```python
from build123d import *

# Parameters (mm, degrees)
SKETCH2_W           = 40
SKETCH2_H           = 34
BOSS_EXTRUDE1_DEPTH = 3.75
SKETCH3_W           = 49.149
SKETCH3_H           = 41.783
BOSS_EXTRUDE2_DEPTH = 1.016
CUT_EXTRUDE1_REACH  = 34.524
SKETCH4_R           = 1.6383
FILLET1_R           = 2.159
CUT_EXTRUDE2_REACH  = 34.524
SKETCH5_R           = 0.649719702
SKETCH6_W           = 36
SKETCH6_H           = 26
CUT_EXTRUDE3_DEPTH  = 0.1016
FILLET2_R           = 3
FILLET3_R           = 1
FILLET4_R           = 1


with BuildPart() as part:
    # Sketch2 → Boss-Extrude1 (new body)
    with BuildSketch(Plane(origin=(0, 0, 0), x_dir=(1, 0, 0), z_dir=(0, 1, 0))):
        Rectangle(SKETCH2_W, SKETCH2_H)
    extrude(amount=BOSS_EXTRUDE1_DEPTH)

    # Sketch3 → Boss-Extrude2 (add)
    with BuildSketch(Plane(origin=(0, 0, 0), x_dir=(1, 0, 0), z_dir=(0, 1, 0))):
        with Locations((0, -0.0815)):
            Rectangle(SKETCH3_W, SKETCH3_H)
    extrude(amount=-BOSS_EXTRUDE2_DEPTH)

    # Sketch4 → Cut-Extrude1 (cut, up to next)
    with BuildSketch(Plane(origin=(0, 0, 0), x_dir=(1, 0, 0), z_dir=(0, 1, 0)), mode=Mode.PRIVATE) as cut_extrude1_sk1:
        with Locations(Location((-22.5, 18.5, 0), (0, 0, 270))):
            Circle(SKETCH4_R)
    cut_extrude1_tool1 = extrude(cut_extrude1_sk1.sketch, amount=-CUT_EXTRUDE1_REACH, mode=Mode.PRIVATE) & part.part
    # Sketch4 → Cut-Extrude1 (cut, up to next)
    with BuildSketch(Plane(origin=(0, 0, 0), x_dir=(1, 0, 0), z_dir=(0, 1, 0)), mode=Mode.PRIVATE) as cut_extrude1_sk2:
        with Locations(Location((-22.5, -18.5, 0), (0, 0, 270))):
            Circle(SKETCH4_R)
    cut_extrude1_tool2 = extrude(cut_extrude1_sk2.sketch, amount=-CUT_EXTRUDE1_REACH, mode=Mode.PRIVATE) & part.part
    # Sketch4 → Cut-Extrude1 (cut, up to next)
    with BuildSketch(Plane(origin=(0, 0, 0), x_dir=(1, 0, 0), z_dir=(0, 1, 0)), mode=Mode.PRIVATE) as cut_extrude1_sk3:
        with Locations(Location((22.5, 18.5, 0), (0, 0, 270))):
            Circle(SKETCH4_R)
    cut_extrude1_tool3 = extrude(cut_extrude1_sk3.sketch, amount=-CUT_EXTRUDE1_REACH, mode=Mode.PRIVATE) & part.part
    # Sketch4 → Cut-Extrude1 (cut, up to next)
    with BuildSketch(Plane(origin=(0, 0, 0), x_dir=(1, 0, 0), z_dir=(0, 1, 0)), mode=Mode.PRIVATE) as cut_extrude1_sk4:
        with Locations(Location((22.5, -18.5, 0), (0, 0, 270))):
            Circle(SKETCH4_R)
    cut_extrude1_tool4 = extrude(cut_extrude1_sk4.sketch, amount=-CUT_EXTRUDE1_REACH, mode=Mode.PRIVATE) & part.part
    add(cut_extrude1_tool1.solids().sort_by_distance((-22.5, 0, -18.5))[0], mode=Mode.SUBTRACT)
    add(cut_extrude1_tool2.solids().sort_by_distance((-22.5, 0, 18.5))[0], mode=Mode.SUBTRACT)
    add(cut_extrude1_tool3.solids().sort_by_distance((22.5, 0, -18.5))[0], mode=Mode.SUBTRACT)
    add(cut_extrude1_tool4.solids().sort_by_distance((22.5, 0, 18.5))[0], mode=Mode.SUBTRACT)

    # Fillet1
    fillet1_edges = [part.edges().sort_by_distance(p)[0] for p in [
        (-24.5745, -0.508, 20.973),
        (-24.5745, -0.508, -20.81),
        (24.5745, -0.508, -20.81),
        (24.5745, -0.508, 20.973),
    ]]
    fillet(fillet1_edges, radius=FILLET1_R)

    # Sketch5 → Cut-Extrude2 (cut, up to next)
    with BuildSketch(Plane(origin=(0, 0, 0), x_dir=(1, 0, 0), z_dir=(0, 1, 0)), mode=Mode.PRIVATE) as cut_extrude2_sk1:
        with Locations(Location((-1.27, 19.2225, 0), (0, 0, 270))):
            Circle(SKETCH5_R)
    cut_extrude2_tool1 = extrude(cut_extrude2_sk1.sketch, amount=-CUT_EXTRUDE2_REACH, mode=Mode.PRIVATE) & part.part
    # Sketch5 → Cut-Extrude2 (cut, up to next)
    with BuildSketch(Plane(origin=(0, 0, 0), x_dir=(1, 0, 0), z_dir=(0, 1, 0)), mode=Mode.PRIVATE) as cut_extrude2_sk2:
        with Locations(Location((-3.81, 19.2225, 0), (0, 0, 270))):
            Circle(SKETCH5_R)
    cut_extrude2_tool2 = extrude(cut_extrude2_sk2.sketch, amount=-CUT_EXTRUDE2_REACH, mode=Mode.PRIVATE) & part.part
    # Sketch5 → Cut-Extrude2 (cut, up to next)
    with BuildSketch(Plane(origin=(0, 0, 0), x_dir=(1, 0, 0), z_dir=(0, 1, 0)), mode=Mode.PRIVATE) as cut_extrude2_sk3:
        with Locations(Location((-6.35, 19.2225, 0), (0, 0, 270))):
            Circle(SKETCH5_R)
    cut_extrude2_tool3 = extrude(cut_extrude2_sk3.sketch, amount=-CUT_EXTRUDE2_REACH, mode=Mode.PRIVATE) & part.part
    # Sketch5 → Cut-Extrude2 (cut, up to next)
    with BuildSketch(Plane(origin=(0, 0, 0), x_dir=(1, 0, 0), z_dir=(0, 1, 0)), mode=Mode.PRIVATE) as cut_extrude2_sk4:
        with Locations(Location((1.27, 19.2225, 0), (0, 0, 270))):
            Circle(SKETCH5_R)
    cut_extrude2_tool4 = extrude(cut_extrude2_sk4.sketch, amount=-CUT_EXTRUDE2_REACH, mode=Mode.PRIVATE) & part.part
    # Sketch5 → Cut-Extrude2 (cut, up to next)
    with BuildSketch(Plane(origin=(0, 0, 0), x_dir=(1, 0, 0), z_dir=(0, 1, 0)), mode=Mode.PRIVATE) as cut_extrude2_sk5:
        with Locations(Location((3.81, 19.2225, 0), (0, 0, 270))):
            Circle(SKETCH5_R)
    cut_extrude2_tool5 = extrude(cut_extrude2_sk5.sketch, amount=-CUT_EXTRUDE2_REACH, mode=Mode.PRIVATE) & part.part
    # Sketch5 → Cut-Extrude2 (cut, up to next)
    with BuildSketch(Plane(origin=(0, 0, 0), x_dir=(1, 0, 0), z_dir=(0, 1, 0)), mode=Mode.PRIVATE) as cut_extrude2_sk6:
        with Locations(Location((6.35, 19.2225, 0), (0, 0, 270))):
            Circle(SKETCH5_R)
    cut_extrude2_tool6 = extrude(cut_extrude2_sk6.sketch, amount=-CUT_EXTRUDE2_REACH, mode=Mode.PRIVATE) & part.part
    # Sketch5 → Cut-Extrude2 (cut, up to next)
    with BuildSketch(Plane(origin=(0, 0, 0), x_dir=(1, 0, 0), z_dir=(0, 1, 0)), mode=Mode.PRIVATE) as cut_extrude2_sk7:
        with Locations(Location((6.35, -18.687, 0), (0, 0, 90))):
            Circle(SKETCH5_R)
    cut_extrude2_tool7 = extrude(cut_extrude2_sk7.sketch, amount=-CUT_EXTRUDE2_REACH, mode=Mode.PRIVATE) & part.part
    # Sketch5 → Cut-Extrude2 (cut, up to next)
    with BuildSketch(Plane(origin=(0, 0, 0), x_dir=(1, 0, 0), z_dir=(0, 1, 0)), mode=Mode.PRIVATE) as cut_extrude2_sk8:
        with Locations(Location((3.81, -18.687, 0), (0, 0, 90))):
            Circle(SKETCH5_R)
    cut_extrude2_tool8 = extrude(cut_extrude2_sk8.sketch, amount=-CUT_EXTRUDE2_REACH, mode=Mode.PRIVATE) & part.part
    # Sketch5 → Cut-Extrude2 (cut, up to next)
    with BuildSketch(Plane(origin=(0, 0, 0), x_dir=(1, 0, 0), z_dir=(0, 1, 0)), mode=Mode.PRIVATE) as cut_extrude2_sk9:
        with Locations(Location((1.27, -18.687, 0), (0, 0, 90))):
            Circle(SKETCH5_R)
    cut_extrude2_tool9 = extrude(cut_extrude2_sk9.sketch, amount=-CUT_EXTRUDE2_REACH, mode=Mode.PRIVATE) & part.part
    # Sketch5 → Cut-Extrude2 (cut, up to next)
    with BuildSketch(Plane(origin=(0, 0, 0), x_dir=(1, 0, 0), z_dir=(0, 1, 0)), mode=Mode.PRIVATE) as cut_extrude2_sk10:
        with Locations(Location((-6.35, -18.687, 0), (0, 0, 90))):
            Circle(SKETCH5_R)
    cut_extrude2_tool10 = extrude(cut_extrude2_sk10.sketch, amount=-CUT_EXTRUDE2_REACH, mode=Mode.PRIVATE) & part.part
    # Sketch5 → Cut-Extrude2 (cut, up to next)
    with BuildSketch(Plane(origin=(0, 0, 0), x_dir=(1, 0, 0), z_dir=(0, 1, 0)), mode=Mode.PRIVATE) as cut_extrude2_sk11:
        with Locations(Location((-3.81, -18.687, 0), (0, 0, 90))):
            Circle(SKETCH5_R)
    cut_extrude2_tool11 = extrude(cut_extrude2_sk11.sketch, amount=-CUT_EXTRUDE2_REACH, mode=Mode.PRIVATE) & part.part
    # Sketch5 → Cut-Extrude2 (cut, up to next)
    with BuildSketch(Plane(origin=(0, 0, 0), x_dir=(1, 0, 0), z_dir=(0, 1, 0)), mode=Mode.PRIVATE) as cut_extrude2_sk12:
        with Locations(Location((-1.27, -18.687, 0), (0, 0, 90))):
            Circle(SKETCH5_R)
    cut_extrude2_tool12 = extrude(cut_extrude2_sk12.sketch, amount=-CUT_EXTRUDE2_REACH, mode=Mode.PRIVATE) & part.part
    add(cut_extrude2_tool1.solids().sort_by_distance((-1.27, 0, -19.2225))[0], mode=Mode.SUBTRACT)
    add(cut_extrude2_tool2.solids().sort_by_distance((-3.81, 0, -19.2225))[0], mode=Mode.SUBTRACT)
    add(cut_extrude2_tool3.solids().sort_by_distance((-6.35, 0, -19.2225))[0], mode=Mode.SUBTRACT)
    add(cut_extrude2_tool4.solids().sort_by_distance((1.27, 0, -19.2225))[0], mode=Mode.SUBTRACT)
    add(cut_extrude2_tool5.solids().sort_by_distance((3.81, 0, -19.2225))[0], mode=Mode.SUBTRACT)
    add(cut_extrude2_tool6.solids().sort_by_distance((6.35, 0, -19.2225))[0], mode=Mode.SUBTRACT)
    add(cut_extrude2_tool7.solids().sort_by_distance((6.35, 0, 18.687))[0], mode=Mode.SUBTRACT)
    add(cut_extrude2_tool8.solids().sort_by_distance((3.81, 0, 18.687))[0], mode=Mode.SUBTRACT)
    add(cut_extrude2_tool9.solids().sort_by_distance((1.27, 0, 18.687))[0], mode=Mode.SUBTRACT)
    add(cut_extrude2_tool10.solids().sort_by_distance((-6.35, 0, 18.687))[0], mode=Mode.SUBTRACT)
    add(cut_extrude2_tool11.solids().sort_by_distance((-3.81, 0, 18.687))[0], mode=Mode.SUBTRACT)
    add(cut_extrude2_tool12.solids().sort_by_distance((-1.27, 0, 18.687))[0], mode=Mode.SUBTRACT)

    # Sketch6 → Cut-Extrude3 (cut)
    with BuildSketch(Plane(origin=(0, 3.75, 0), x_dir=(1, 0, 0), z_dir=(0, 1, 0))):
        with Locations((0, 2.75)):
            Rectangle(SKETCH6_W, SKETCH6_H)
    extrude(amount=-CUT_EXTRUDE3_DEPTH, mode=Mode.SUBTRACT)

    # Fillet2
    fillet2_edges = [part.edges().sort_by_distance(p)[0] for p in [
        (-18, 3.6992, 10.25),
        (-18, 3.6992, -15.75),
        (18, 3.6992, -15.75),
        (18, 3.6992, 10.25),
    ]]
    fillet(fillet2_edges, radius=FILLET2_R)

    # Fillet3
    fillet3_edges = [part.edges().sort_by_distance(p)[0] for p in [
        (-20, 1.875, -17),
        (20, 1.875, -17),
        (20, 1.875, 17),
        (-20, 1.875, 17),
    ]]
    fillet(fillet3_edges, radius=FILLET3_R)

    # Fillet4
    fillet4_edges = [part.edges().sort_by_distance(p)[0] for p in [
        (-20, 3.75, 0),
        (0, 3.75, -17),
        (0, 3.75, 17),
        (20, 3.75, 0),
        (19.707106781, 3.75, -16.707106781),
        (19.707106781, 3.75, 16.707106781),
        (-19.707106781, 3.75, 16.707106781),
        (-19.707106781, 3.75, -16.707106781),
    ]]
    fillet(fillet4_edges, radius=FILLET4_R)


solid = part.part
```
Can you work these out from the model? Positions are in its coordinate system, mm. A direction names the side the tool comes from. Give positions to 0.01 mm unless a question says otherwise; leave off trailing zeros. Write each loop counter-clockwise with the first axis right and the second up, starting at its lowest first coordinate (ties: lowest second). Pieces come first, ordered by that corner, then holes. Notation, with made-up numbers: (54.25, 23.5) -> (78.25, 23.5) arc R26 ccw to (78.25, 51.5) -> close; hole circle Ø6 at (84, -17). An arc over 180 degrees is marked (long way). One line per item, written item: value.
Q1. We'd pull the mould along X, two halves only. Please class faces 4 (the face through (-0.3, -0.5, -20.81)), 5 (the face through (-23.95, -0.5, 19.26)), 6 (the face through (19.699, 3.465, 0.224)): +X half, -X half, draft (parallel to the pull), parting line (faces both ways), or undercut.
Results found:
face 4: draft
face 5: undercut
face 6: +X half
Q2. Which directions (+Z, -Z, +X, -X, +Y, -Y) give clear straight access to the entire face, cutting with the end or side of a thin tool? Please do faces 1 (the face through (20, 1, 0)), 2 (the face through (-19.715, 1.394, 16.699)), 3 (the face through (-19.715, 1.394, -16.699)).
Results found:
face 1: +Z, -Z, +X, +Y
face 2: +Z, -X, +Y
face 3: -Z, -X, +Y
Q3. Please list where these lines run through material, in increasing order: line 1 (X direction, y = -0.8, z = -18.5); line 2 (X direction, y = 1.05, z = -12.5); line 3 (Y direction, x = -7.5, z = -5). Write a range as [from, to].
Results found:
line 1: x = [-24.57, -24.14], [-20.86, 20.86], [24.14, 24.57]
line 2: x = [-20, 20]
line 3: y = [-1.02, 3.65]
Q4. Imagine slicing it at B-B on y = 1. Please give me the cut outline in (x, z), and give its area (3 significant figures).
Results found:
outline: (-20, -16) arc R1 ccw to (-19, -17) -> (19, -17) arc R1 ccw to (20, -16) -> (20, 16) arc R1 ccw to (19, 17) -> (-19, 17) arc R1 ccw to (-20, 16) -> close
area: 1,360 mm^2
Q5. Imagine slicing it at D-D on z = -11. Please give me the cut outline in (x, y), and give its area (3 significant figures).
Results found:
outline: (-24.57, -1.02) -> (24.57, -1.02) -> (24.57, 0) -> (20, 0) -> (20, 2.75) arc R1 ccw to (19, 3.75) -> (18, 3.75) -> (18, 3.65) -> (-18, 3.65) -> (-18, 3.75) -> (-19, 3.75) arc R1 ccw to (-20, 2.75) -> (-20, 0) -> (-24.57, 0) -> close
area: 196 mm^2
Q6. Imagine slicing it at A-A on x = -6.35. Please give me the cut outline in (y, z).
Results found:
outline: (-1.02, -20.81) -> (0, -20.81) -> (0, -19.87) -> (-1.02, -19.87) -> close; (-1.02, -18.57) -> (0, -18.57) -> (0, -17) -> (2.75, -17) arc R1 ccw to (3.75, -16) -> (3.75, -15.75) -> (3.65, -15.75) -> (3.65, 10.25) -> (3.75, 10.25) -> (3.75, 16) arc R1 ccw to (2.75, 17) -> (0, 17) -> (0, 18.04) -> (-1.02, 18.04) -> close; (-1.02, 19.34) -> (0, 19.34) -> (0, 20.97) -> (-1.02, 20.97) -> close
Q7. For P1, Ø1, axis at x = 5.5, z = 2, coming from the +Y side; P2, Ø1.5, axis at x = -1.27, z = -19.22, coming from the +Y side; P3, Ø2, axis at y = 1.5, z = -16.5, coming from the -X side, each with a flat end and sliding along its axis, tell me the tip position at first contact or that it passes through.
Results found:
P1: stops at y = 3.65
P2: stops at y = 0
P3: stops at x = -20
Q8. Imagine slicing it at C-C on x = 5. Please give me the cut outline in (y, z).
Results found:
outline: (-1.02, -20.81) -> (0, -20.81) -> (0, -17) -> (2.75, -17) arc R1 ccw to (3.75, -16) -> (3.75, -15.75) -> (3.65, -15.75) -> (3.65, 10.25) -> (3.75, 10.25) -> (3.75, 16) arc R1 ccw to (2.75, 17) -> (0, 17) -> (0, 20.97) -> (-1.02, 20.97) -> close
